Autodesk Inventor part; units mm, degrees
ref_plane "YZ Plane" through (0, 0, 0) normal (1, 0, 0) x (0, 1, 0)
ref_plane "XZ Plane" through (0, 0, 0) normal (0, 1, 0) x (-1, 0, 0)
ref_plane "XY Plane" through (0, 0, 0) normal (0, 0, 1) x (1, 0, 0)
sketch "Sketch1" plane through (0, 0, 0) normal (0, 1, 0) x (-1, 0, 0)
  line L0 (7, 21) -> (-7, 21)
  line L1 (-11, 17) -> (-11, -17)
  line L2 (-7, -21) -> (7, -21)
  line L3 (11, -17) -> (11, 17)
  line L4 (6, 3.6056) -> (6, -3.6056)
  line L5 (-6, -3.6056) -> (-6, 3.6056)
  line L6 (6.364, 6.364) -> (-6.364, 6.364) construction
  line L7 (-6.364, 6.364) -> (-6.364, -6.364) construction
  line L8 (-6.364, -6.364) -> (6.364, -6.364) construction
  line L9 (6.364, -6.364) -> (6.364, 6.364) construction
  arc A0 (-6, -3.6056) -> (6, -3.6056) centre (0, 0) ccw
  arc A1 (6, 3.6056) -> (-6, 3.6056) centre (0, 0) ccw
  arc A2 (-11, -17) -> (-7, -21) centre (-7, -17) ccw
  arc A3 (-7, 21) -> (-11, 17) centre (-7, 17) ccw
  arc A4 (11, 17) -> (7, 21) centre (7, 17) ccw
  arc A5 (7, -21) -> (11, -17) centre (7, -17) ccw
  point P0 (0, -21)
  point P1 (0, -7)
  point P2 (6.364, 0)
  point P3 (11, 0)
  point P4 (6, 0)
  point P5 (0, -6.364)
  dimension "d0" = 7
  dimension "d1" = 12
  dimension "d2" = 18
  dimension "d3" = 22
  dimension "d4" = 42
  dimension "d5" = 4
extrude "Extrusion1" add sketch "Sketch1" against normal blind 3
hole "Hole1" at (-7, 0, 17) at (7, 0, 17) at (7, 0, -17) at (-7, 0, -17) direction (0, -1, 0) diameter 3 end through all
hole "Hole2" at (-6.364, 0, -6.364) at (6.364, 0, -6.364) at (6.364, 0, 6.364) at (-6.364, 0, 6.364) direction (0, -1, 0) diameter 2 end through all
properties part number "motor_plate"
Verification items for the finished model (mm, model axes). A direction names the side the tool comes from. Coordinates: 2 decimals unless noted, no trailing zeros. Loops run counter-clockwise (first coordinate to the right, second up) from the corner with the lowest first, then second, coordinate; pieces in that order, holes last. Notation, with made-up numbers: (71.25, -9.5) -> (102.25, -9.5) arc R12 ccw to (102.25, 5.5) -> close; hole circle Ø8 at (41, 37.5). An arc over 180 degrees is marked (long way). Answer in a Markdown table with one row per item. Add a question column.
1. Material ranges on probe 1 along X at (y, z) = (-1.05, 17); probe 2 along Z at (x, y) = (8, -0.7); probe 3 along Z at (x, y) = (7.75, -2.2), recorded low to high. Write a range as [from, to].
2. Section check C-C, the plane y = -2.35. Give the number of separate pieces and of enclosed holes in the cut face, then the cut area to 3 significant figures.
3. Section check A-A, the plane z = 0. Enter the section's corners in (x, y).
4. Section check B-B, the plane z = 16. Enter the section's corners in (x, y).
5. Section check D-D, the plane x = -9. Enter the section's corners in (y, z).
6. Draft check along X on faces 3 (the face through (9.797, -1.479, 19.859)), 4 (the face through (7.9, -1.5, 15.8)), 5 (the face through (0, -1, 21)). Enter one of: +X half, -X half, draft (parallel to the pull), parting line (faces both ways), or undercut.
7. Access from +Z, -Z, +X, -X, +Y, -Y to the whole of each face (thin tool, end or side, straight path). Record for faces 1 (the face through (7, 0, 0)), 2 (the face through (-6, -1, 0)).
Derived:
| question | item | result |
|---|---|---|
| 1 | probe 1 | x = [-11, -8.5], [-5.5, 5.5], [8.5, 11] |
| 1 | probe 2 | z = [-20.87, -18.12], [-15.88, 15.88], [18.12, 20.87] |
| 1 | probe 3 | z = [-20.93, -18.3], [-15.7, 15.7], [18.3, 20.93] |
| 2 | separate pieces | 1 |
| 2 | enclosed holes | 9 |
| 2 | area | 725 mm² |
| 3 | outline | (-11, -3) -> (-6, -3) -> (-6, 0) -> (-11, 0) -> close; (6, -3) -> (11, -3) -> (11, 0) -> (6, 0) -> close |
| 4 | outline | (-11, -3) -> (-8.12, -3) -> (-8.12, 0) -> (-11, 0) -> close; (-5.88, -3) -> (5.88, -3) -> (5.88, 0) -> (-5.88, 0) -> close; (8.12, -3) -> (11, -3) -> (11, 0) -> (8.12, 0) -> close |
| 5 | outline | (-3, -20.46) -> (0, -20.46) -> (0, 20.46) -> (-3, 20.46) -> close |
| 6 | face 3 | +X half |
| 6 | face 4 | undercut |
| 6 | face 5 | draft |
| 7 | face 1 | +Z, -Z, +X, -X, +Y |
| 7 | face 2 | +Y, -Y |
